Verification items for the finished model (mm, model axes). A direction names the side the tool comes from. Round coordinates to 2 decimals unless told otherwise and drop trailing zeros. Write each loop counter-clockwise with the first axis right and the second up, starting at its lowest first coordinate (ties: lowest second). Pieces come first, ordered by that corner, then holes. Notation, with made-up numbers: M 21,-18 L 66,-18 A16 cw 66,2 Z; hole C 34.5,45.5 d5. An arc over 180 degrees is marked long. One line per item, written item: value. Start each with the question number.
from build123d import *

# Parameters (mm, degrees)
SKETCH1_W                = 240
SKETCH1_H                = 30
SKETCH1_W_2              = 12.7
SKETCH1_H_2              = 12.7
BOSS_EXTRUDE1_DEPTH      = 4
SKETCH2_W                = 12.7
SKETCH2_H                = 12.7
BOSS_EXTRUDE2_DEPTH      = 13
BOSS_EXTRUDE2_DEPTH_BACK = 4
SKETCH3_W                = 217.126937851
SKETCH3_H                = 95.437848018
CUT_EXTRUDE1_DEPTH       = 14
CUT_EXTRUDE1_DEPTH_BACK  = 5
FILLET1_R                = 1
CHAMFER1_SIZE            = 0.4
CHAMFER1_SIZE2           = 8


with BuildPart() as part:
    # Sketch1 → Boss-Extrude1 (new body)
    with BuildSketch(Plane(origin=(0, 0, 0), x_dir=(1, 0, 0), z_dir=(0, 1, 0))):
        with Locations((120, 15)):
            Rectangle(SKETCH1_W, SKETCH1_H)
        with Locations((13.25, 15)):
            Rectangle(SKETCH1_W_2, SKETCH1_H_2, mode=Mode.SUBTRACT)
        with Locations((43.75, 15)):
            Rectangle(SKETCH1_W_2, SKETCH1_H_2, mode=Mode.SUBTRACT)
        with Locations((74.25, 15)):
            Rectangle(SKETCH1_W_2, SKETCH1_H_2, mode=Mode.SUBTRACT)
        with Locations((104.75, 15)):
            Rectangle(SKETCH1_W_2, SKETCH1_H_2, mode=Mode.SUBTRACT)
        with Locations((135.25, 15)):
            Rectangle(SKETCH1_W_2, SKETCH1_H_2, mode=Mode.SUBTRACT)
        with Locations((165.75, 15)):
            Rectangle(SKETCH1_W_2, SKETCH1_H_2, mode=Mode.SUBTRACT)
        with Locations((196.25, 15)):
            Rectangle(SKETCH1_W_2, SKETCH1_H_2, mode=Mode.SUBTRACT)
        with Locations((226.75, 15)):
            Rectangle(SKETCH1_W_2, SKETCH1_H_2, mode=Mode.SUBTRACT)
    extrude(amount=BOSS_EXTRUDE1_DEPTH)

    # Sketch2 → Boss-Extrude2 (add, two sides)
    with BuildSketch(Plane(origin=(0, 4, 0), x_dir=(1, 0, 0), z_dir=(0, 1, 0))) as boss_extrude2_sk:
        with Locations((13.25, 15)):
            Rectangle(SKETCH2_W, SKETCH2_H)
        with Locations((43.75, 15)):
            Rectangle(SKETCH2_W, SKETCH2_H)
        with Locations((74.25, 15)):
            Rectangle(SKETCH2_W, SKETCH2_H)
        with Locations((104.75, 15)):
            Rectangle(SKETCH2_W, SKETCH2_H)
        with Locations((135.25, 15)):
            Rectangle(SKETCH2_W, SKETCH2_H)
        with Locations((165.75, 15)):
            Rectangle(SKETCH2_W, SKETCH2_H)
        with Locations((196.25, 15)):
            Rectangle(SKETCH2_W, SKETCH2_H)
        with Locations((226.75, 15)):
            Rectangle(SKETCH2_W, SKETCH2_H)
    extrude(amount=BOSS_EXTRUDE2_DEPTH)
    extrude(boss_extrude2_sk.sketch, amount=-BOSS_EXTRUDE2_DEPTH_BACK)

    # Sketch3 → Cut-Extrude1 (cut, two sides)
    with BuildSketch(Plane(origin=(0, 4, 0), x_dir=(1, 0, 0), z_dir=(0, 1, 0))) as cut_extrude1_sk:
        with Locations((136.509114297, 10.683129124)):
            Rectangle(SKETCH3_W, SKETCH3_H)
    extrude(amount=CUT_EXTRUDE1_DEPTH, mode=Mode.SUBTRACT)
    extrude(cut_extrude1_sk.sketch, amount=-CUT_EXTRUDE1_DEPTH_BACK, mode=Mode.SUBTRACT)

    # Fillet1
    fillet1_edges = [part.edges().sort_by_distance(p)[0] for p in [
        (6.9, 17, -15),
        (13.25, 17, -8.65),
        (19.6, 17, -15),
        (13.25, 17, -21.35),
    ]]
    fillet(fillet1_edges, radius=FILLET1_R)

    # Chamfer1
    chamfer1_edges = [part.edges().sort_by_distance(p)[0] for p in [
        (6.9, 4, -15),
        (13.25, 4, -8.65),
        (19.6, 4, -15),
        (13.25, 4, -21.35),
    ]]
    chamfer1_side = [part.faces().sort_by_distance(p)[0] for p in [
        (0.409995012, 4, -15),
    ]]
    chamfer(chamfer1_edges, length=CHAMFER1_SIZE, length2=CHAMFER1_SIZE2, reference=chamfer1_side[0])


solid = part.part
1) Cross-section at D-D (z = -24). Record the boundary of the cut face in (x, y), then the cut area to 3 significant figures.
2) Access from +Z, -Z, +X, -X, +Y, -Y to the whole of each face (thin tool, end or side, straight path). Record for faces 1 (the flat face through (6.9, 14, -15)), 2 (the flat face through (13, 14, -21.35)), 3 (the flat face through (19.6, 14, -15)), 4 (the flat face through (13, 14, -8.65)), 5 (the flat face through (14, 4, -22)).
3) Gauge pin test, flat ends, axial feed: pin 1 Ø3 at (x, y) = (14, 13.5) entering from -Z; pin 2 Ø4 at (y, z) = (6.5, -12) entering from -X (3 decimals); pin 3 Ø3 at (y, z) = (14.5, -17) entering from -X. Record the tip position at first contact, or that the pin passes through.
4) Thickness scan on line 1 (Z direction, x = 12, y = 14.25); line 2 (Y direction, x = 6.25, z = -22.75); line 3 (X direction, y = 12.5, z = -21). Record the ranges inside material, lowest first.
5) Cross-section at B-B (z = -15). Record the boundary of the cut face in (x, y), then the cut area to 3 significant figures.
6) Cross-section at C-C (y = 5). Record the boundary of the cut face in (x, z), then the cut area to 3 significant figures.
7) Cross-section at A-A (x = 10.75). Record the boundary of the cut face in (y, z), then the cut area to 3 significant figures.
Results below:
1. outline: M 0,0 L 27.95,0 L 27.95,4 L 0,4 Z
1. area: 112 mm²
2. face 1: +Z, -Z, -X, +Y
2. face 2: -Z, +X, -X, +Y
2. face 3: +Z, -Z, +X, +Y
2. face 4: +Z, +X, -X, +Y
2. face 5: +Y
3. pin 1: stops at z = -21.35
3. pin 2: stops at x = 6.525
3. pin 3: stops at x = 6.9
4. line 1: z = -21.35 to -8.65
4. line 2: y = 0 to 4
4. line 3: x = 6.9 to 19.6
5. outline: M 0,0 L 27.95,0 L 27.95,4 L 20,4 L 19.6,12 L 19.6,16 A1 ccw 18.6,17 L 7.9,17 A1 ccw 6.9,16 L 6.9,12 L 6.5,4 L 0,4 Z
5. area: 280 mm²
6. outline: M 6.55,-21.7 L 19.95,-21.7 L 19.95,-8.3 L 6.55,-8.3 Z
6. area: 180 mm²
7. outline: M 0,-30 L 4,-30 L 4,-21.75 L 12,-21.35 L 16,-21.35 A1 ccw 17,-20.35 L 17,-9.65 A1 ccw 16,-8.65 L 12,-8.65 L 4,-8.25 L 4,0 L 0,0 Z
7. area: 288 mm²
